Source: CAD feature listing. Evaluate the final solid. Frame: model axes, mm. Give positions to 0.01 mm unless a question says otherwise; leave off trailing zeros. Order: outer loops, then holes, each group sorted by start corner. A loop starts at its lowest first (then second) coordinate and runs counter-clockwise, first axis right, second up. Notation, with made-up numbers: M 83.25,49 L 95.25,49 A15 cw 95.25,66 Z; hole C 24,53.5 d11. An arc over 180 degrees is marked long. Answer in a Markdown table with one row per item. Add a question column.
(1) Pin query (flat end, axial travel): P1, Ø1.5, axis at y = -2, z = -2, coming from the -X side. Return the tip coordinate at first contact, or that it passes through.
(2) Material intervals for line 1 along Y through (x, z) = (4, 2.5); line 2 along Z through (x, y) = (-1.75, 1.75); line 3 along X through (y, z) = (0.5, -4), sorted ascending.
(3) Section query A-A, the plane y = 0.7. Return loops of the section in (x, z) (1 decimal).
from build123d import *

# Parameters (mm, degrees)
F0_R     = 4.7625
F1_DEPTH = 1.5
F2_R     = 4.7625
F3_DEPTH = 1.5
F4_R     = 0.35


with BuildPart() as f1:
    # F0 (on Front) → F1 (new body, symmetric)
    with BuildSketch(Plane.XZ):
        Circle(F0_R)
    extrude(amount=F1_DEPTH, both=True)

    # F2 (on face) → F3 (join)
    with BuildSketch(Plane.XZ.offset(1.5)):
        Circle(F2_R)
    extrude(amount=F3_DEPTH)

    # F4
    f4_edges = [f1.edges().sort_by_distance(p)[0] for p in [
        (-4.7625, -3, 0),
    ]]
    fillet(f4_edges, radius=F4_R)

    # F5: F1 across plane


with BuildPart() as f1_1:
    add(f1.part)
    add(f1.part.mirror(Plane.XZ))


solid = f1_1.part
Values follow:
| question | item | result |
|---|---|---|
| 1 | P1 | stops at x = -4.6 |
| 2 | line 1 | y = -2.82 to 2.82 |
| 2 | line 2 | z = -4.43 to 4.43 |
| 2 | line 3 | x = -2.58 to 2.58 |
| 3 | outline | C 0,0 d9.5 |
